```python
from build123d import *

# Parameters (mm, degrees)
SKETCH1_R           = 3.5
BOSS_EXTRUDE1_DEPTH = 20
SKETCH2_R           = 4.7
BOSS_EXTRUDE2_DEPTH = 10
SKETCH3_R           = 3.5
BOSS_EXTRUDE3_DEPTH = 15
FILLET1_R           = 1
CHAMFER1_SIZE       = 0.5


with BuildPart() as part:
    # Sketch1 → Boss-Extrude1 (new body)
    with BuildSketch(Plane(origin=(0, 0, 0), x_dir=(1, 0, 0), z_dir=(0, 1, 0))):
        Circle(SKETCH1_R)
    extrude(amount=BOSS_EXTRUDE1_DEPTH)

    # Sketch2 → Boss-Extrude2 (add)
    with BuildSketch(Plane(origin=(0, 20, 0), x_dir=(1, 0, 0), z_dir=(0, 1, 0))):
        Circle(SKETCH2_R)
    extrude(amount=BOSS_EXTRUDE2_DEPTH)

    # Sketch3 → Boss-Extrude3 (add)
    with BuildSketch(Plane(origin=(0, 30, 0), x_dir=(1, 0, 0), z_dir=(0, 1, 0))):
        Circle(SKETCH3_R)
    extrude(amount=BOSS_EXTRUDE3_DEPTH)

    # Fillet1
    fillet1_edges = [part.edges().sort_by_distance(p)[0] for p in [
        (-3.5, 30, 0),
        (-3.5, 20, 0),
    ]]
    fillet(fillet1_edges, radius=FILLET1_R)

    # Chamfer1
    chamfer1_edges = [part.edges().sort_by_distance(p)[0] for p in [
        (-3.5, 45, 0),
        (-3.5, 0, 0),
    ]]
    chamfer(chamfer1_edges, length=CHAMFER1_SIZE)


solid = part.part
```
Read the model definition and answer for the solid it produces. Units are mm, in the model's axes. A direction names the side the tool comes from. Give positions to 0.01 mm unless a question says otherwise; leave off trailing zeros. Write each loop counter-clockwise with the first axis right and the second up, starting at its lowest first coordinate (ties: lowest second). Pieces come first, ordered by that corner, then holes. Notation, with made-up numbers: (-20.5, 46) -> (-8.5, 46) arc R28 ccw to (-8.5, 65) -> close; hole circle Ø10 at (-33.5, 30.25). An arc over 180 degrees is marked (long way). Answer in a Markdown table with one row per item.
1) Each of these flat-tipped pins is pushed along its axis until it touches: pin 1 Ø1.5 at (y, z) = (39.5, -3.5) entering from -X; pin 2 Ø4 at (x, y) = (0.5, 8.5) entering from -Z; pin 3 Ø3 at (y, z) = (11, 2) entering from +X. Where does it stop, or does it pass through?
Results list:
| item | result |
|---|---|
| pin 1 | x = -2.17 |
| pin 2 | z = -3.5 |
| pin 3 | x = 3.46 |
2) Straight lines are drawn through the part: line 1 (Y direction, x = 3.25, z = 3); line 2 (Z direction, x = -0.25, y = 3); line 3 (X direction, y = 36.5, z = -3). For each, find the intervals that lie inside material, in ascending order. Write a range as [from, to].
Results list:
| item | result |
|---|---|
| line 1 | [20, 30] |
| line 2 | [-3.49, 3.49] |
| line 3 | [-1.8, 1.8] |
3) Section D-D on y = 33.5 is taken. Give the vertices of the cut face in (x, z), plus the area to 3 significant figures.
Results list:
| item | result |
|---|---|
| outline | circle Ø7 at (0, 0) |
| area | 38.5 mm^2 |
4) Section A-A on z = 0 is taken. Give the vertices of the cut face in (x, y), plus the area to 3 significant figures.
Results list:
| item | result |
|---|---|
| outline | (-4.7, 20) -> (-4.5, 20) arc R1 cw to (-3.5, 19) -> (-3.5, 0.5) -> (-3, 0) -> (3, 0) -> (3.5, 0.5) -> (3.5, 19) arc R1 cw to (4.5, 20) -> (4.7, 20) -> (4.7, 30) -> (4.5, 30) arc R1 cw to (3.5, 31) -> (3.5, 44.5) -> (3, 45) -> (-3, 45) -> (-3.5, 44.5) -> (-3.5, 31) arc R1 cw to (-4.5, 30) -> (-4.7, 30) -> close |
| area | 339 mm^2 |
5) Section C-C on y = 25.5 is taken. Give the vertices of the cut face in (x, z), plus the area to 3 significant figures.
Results list:
| item | result |
|---|---|
| outline | circle Ø9.4 at (0, 0) |
| area | 69.4 mm^2 |
6) A tool of negligible diameter and unlimited length cuts with its end or side. For faces 1 (the cylindrical face through (3.233, 37.656, 1.341)), 2 (the flat face through (0, 0, 0)), 3 (the cylindrical face through (3.233, 9.62, 1.341)), from which of +Z, -Z, +X, -X, +Y, -Y can it reach the whole face along a straight path? Write none if from no direction.
Results list:
| item | result |
|---|---|
| face 1 | +Y |
| face 2 | +Z, -Z, +X, -X, -Y |
| face 3 | -Y |
7) Section B-B on x = 0 is taken. Give the vertices of the cut face in (y, z).
Results list:
| item | result |
|---|---|
| outline | (0, -3) -> (0.5, -3.5) -> (19, -3.5) arc R1 cw to (20, -4.5) -> (20, -4.7) -> (30, -4.7) -> (30, -4.5) arc R1 cw to (31, -3.5) -> (44.5, -3.5) -> (45, -3) -> (45, 3) -> (44.5, 3.5) -> (31, 3.5) arc R1 cw to (30, 4.5) -> (30, 4.7) -> (20, 4.7) -> (20, 4.5) arc R1 cw to (19, 3.5) -> (0.5, 3.5) -> (0, 3) -> close |
